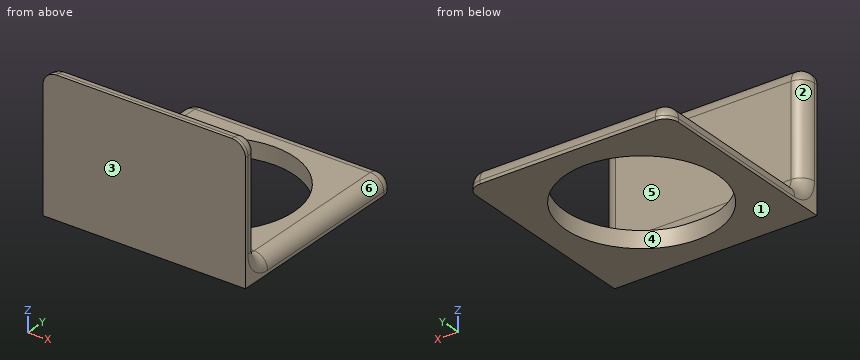
from build123d import *

# Parameters (mm, degrees)
SKETCH2_W           = 38.1
SKETCH2_H           = 38.1
BOSS_EXTRUDE1_DEPTH = 3.175
SKETCH3_W           = 38.1
SKETCH3_H           = 3.175
BOSS_EXTRUDE2_DEPTH = 22.225
FILLET1_R           = 2.54
SKETCH4_R           = 14.2875
CUT_EXTRUDE1_DEPTH  = 60.56828015


with BuildPart() as part:
    # Sketch2 → Boss-Extrude1 (new body)
    with BuildSketch(Plane.XY):
        with Locations((19.05, 19.05)):
            Rectangle(SKETCH2_W, SKETCH2_H)
    extrude(amount=BOSS_EXTRUDE1_DEPTH)

    # Sketch3 → Boss-Extrude2 (add)
    with BuildSketch(Plane.XY.offset(3.175)):
        with Locations((19.05, 1.5875)):
            Rectangle(SKETCH3_W, SKETCH3_H)
    extrude(amount=BOSS_EXTRUDE2_DEPTH)

    # Fillet1
    fillet1_edges = [part.edges().sort_by_distance(p)[0] for p in [
        (19.05, 38.1, 3.175),
        (38.1, 20.6375, 3.175),
        (0, 3.175, 14.2875),
        (19.05, 3.175, 3.175),
        (38.1, 3.175, 14.2875),
        (0, 1.5875, 25.4),
        (38.1, 1.5875, 25.4),
        (19.05, 3.175, 25.4),
        (0, 20.6375, 3.175),
        (0, 38.1, 1.5875),
        (38.1, 38.1, 1.5875),
    ]]
    fillet(fillet1_edges, radius=FILLET1_R)

    # Sketch4 → Cut-Extrude1 (cut, through all)
    with BuildSketch(Plane(origin=(0, 0, 0), x_dir=(-1, 0, 0), z_dir=(0, 0, -1))):
        with Locations((-19.05, 19.05)):
            Circle(SKETCH4_R)
    extrude(amount=-CUT_EXTRUDE1_DEPTH, mode=Mode.SUBTRACT)


solid = part.part
Read the model definition and answer for the solid it produces. Units are mm, in the model's axes. Face numbers are marked on the shaded views. A direction names the side the tool comes from. Round coordinates to 2 decimals unless told otherwise and drop trailing zeros. Loops run counter-clockwise (first coordinate to the right, second up) from the corner with the lowest first, then second, coordinate; pieces in that order, holes last. Notation, with made-up numbers: (-16, 12.5) - (16, 12.5) arc R21 ccw to (16, 44.5) - close; hole circle Ø2 at (0, 26.25). An arc over 180 degrees is marked (long way). One line per question, with ' | ' between items. Start each with the question number.
Q1. Flat-ended cylindrical pins translate along their axes: pin 1 (8 mm diameter, centred on y = 9.5, z = 20, fed in from +X); pin 2 (10 mm diameter, centred on y = 6, z = 19, fed in from +X); pin 3 (1 mm diameter, centred on x = 19.5, z = 13, fed in from +Y) (3 decimals). Find the tip coordinate at first contact, or state that the pin passes through.
Q2. For the marked faces 5 and 6, determine the directions among +Z, -Z, +X, -X, +Y, -Y from which every point of the face is accessible in a straight line to the end or side of a thin tool.
Q3. Find the intervals of material crossed by L1, parallel to X at y = 19.05, z = 0.85; L2, parallel to Z at x = 6.5, y = 35 (3 decimals), in increasing order.
Q4. Section C-C on z = 15.75 is taken. Give the vertices of the cut face in (x, y) (3 decimals), plus the area to 3 significant figures.
Q5. Section D-D on y = 8 is taken. Give the vertices of the cut face in (x, z) (3 decimals), plus the area to 3 significant figures.
Q6. Section A-A on x = 19.05 is taken. Give the vertices of the cut face in (y, z) (1 decimal).
Q7. Section B-B on y = 19.05 is taken. Give the vertices of the cut face in (x, z) (1 decimal), plus the area to 3 significant figures.
Q8. For a pull along Y with two mould halves and no side action, classify the marked faces 1, 2, 3 and 4 as +Y half, -Y half, draft (parallel to the pull), parting line (faces both ways), or undercut.
Established:
1) pin 1: through | pin 2: x = 38.07 | pin 3: y = 3.175
2) face 5: +Z, +X, -X, +Y | face 6: +Z, +X, +Y
3) L1: 0.01 to 4.76, 33.34 to 38.09 | L2: 0 to 3.175
4) outline: (0, 0) - (38.1, 0) - (38.1, 0.635) arc R2.54 ccw to (35.56, 3.175) - (2.54, 3.175) arc R2.54 ccw to (0, 0.635) - close | area: 118 mm²
5) outline: (0, 0) - (9.993, 0) - (9.993, 3.175) - (2.54, 3.175) arc R2.54 ccw to (0, 0.635) - close; (28.107, 0) - (38.1, 0) - (38.1, 0.635) arc R2.54 ccw to (35.56, 3.175) - (28.107, 3.175) - close | area: 60.7 mm²
6) outline: (0, 0) - (4.8, 0) - (4.8, 3.4) arc R2.5 cw to (3.2, 5.7) - (3.2, 22.9) arc R2.5 ccw to (0.6, 25.4) - (0, 25.4) - close; (33.3, 0) - (38.1, 0) - (38.1, 0.6) arc R2.5 ccw to (35.6, 3.2) - (33.3, 3.2) - close
7) outline: (0, 0) - (4.8, 0) - (4.8, 3.2) - (2.5, 3.2) arc R2.5 ccw to (0, 0.6) - close; (33.3, 0) - (38.1, 0) - (38.1, 0.6) arc R2.5 ccw to (35.6, 3.2) - (33.3, 3.2) - close | area: 27.5 mm²
8) face 1: draft | face 2: +Y half | face 3: -Y half | face 4: undercut
